For this review, use the dimensioned drawing (mm, ordinates from the lowest corner) and the shaded views. A direction names the side the tool comes from. Give positions to 0.01 mm unless a question says otherwise; leave off trailing zeros. Order: outer loops, then holes, each group sorted by start corner. A loop starts at its lowest first (then second) coordinate and runs counter-clockwise, first axis right, second up.
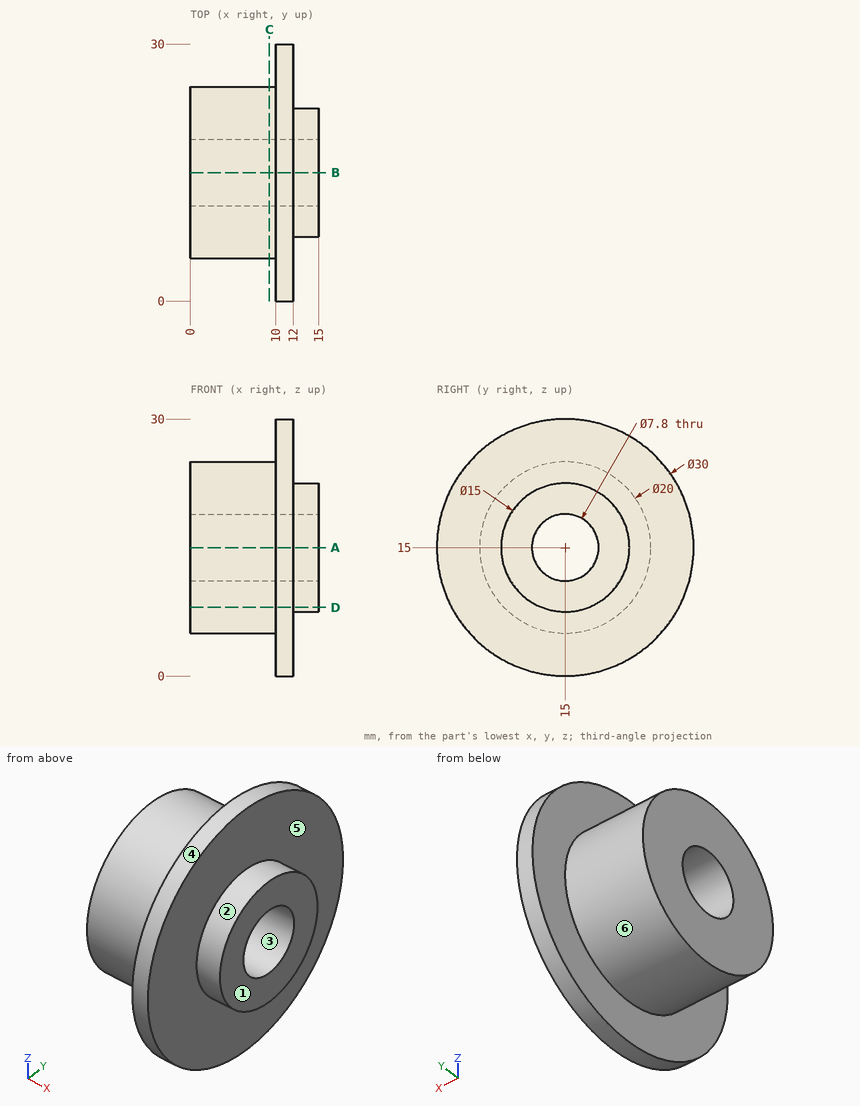
1. Draft analysis for pull direction Z (two halves, no side actions). For the marked faces 1, 2 and 3, state which applies: pulls with the +Z half, pulls with the -Z half, needs draft (parallel to the pull), parting line crosses it, or undercut.
Recorded:
face 1: needs draft
face 2: parting line crosses it
face 3: undercut
2. For line 1 along Z through (x, y) = (3, 15); line 2 along Z through (x, y) = (12.25, 15); line 3 along X through (y, z) = (24.25, 10), list the stretches that pass through material, from the lowest coordinate up.
Recorded:
line 1: z = 5 to 11.1, 18.9 to 25
line 2: z = 7.5 to 11.1, 18.9 to 22.5
line 3: x = 10 to 12
3. Take a section at C-C (x = 9.25). State the section outline as (y, z) points.
Recorded:
outline: circle Ø20 at (15, 15); hole circle Ø7.8 at (15, 15)
4. Machinability: for the marked faces 4, 5 and 6, which of the approach directions +Z, -Z, +X, -X, +Y, -Y give a long, thin tool a straight path to every point of the face, cutting with its end or side? Answer none if there is none.
Recorded:
face 4: +X, -X
face 5: +X
face 6: -X
5. Take a section at D-D (z = 8). State the section outline as (x, y) points, then the cut area to 3 significant figures.
Recorded:
outline: (0, 7.86) - (10, 7.86) - (10, 1.73) - (12, 1.73) - (12, 12.31) - (15, 12.31) - (15, 17.69) - (12, 17.69) - (12, 28.27) - (10, 28.27) - (10, 22.14) - (0, 22.14) - close
area: 212 mm2
6. Take a section at A-A (z = 15). State the section outline as (x, y) points, then the cut area to 3 significant figures.
Recorded:
outline: (0, 5) - (10, 5) - (10, 0) - (12, 0) - (12, 7.5) - (15, 7.5) - (15, 11.1) - (0, 11.1) - close; (0, 18.9) - (15, 18.9) - (15, 22.5) - (12, 22.5) - (12, 30) - (10, 30) - (10, 25) - (0, 25) - close
area: 188 mm2
7. For pin 1 (8 mm diameter, centred on x = 9.5, y = 21.5, fed in from -Z); pin 2 (8 mm diameter, centred on x = 4, z = 27, fed in from -Y); pin 3 (5 mm diameter, centred on x = 4, z = 21, fed in from +Y), all flat-tipped, find the tip position at first contact; note any pin that passes through.
Recorded:
pin 1: stops at z = 0.22
pin 2: stops at y = 9
pin 3: stops at y = 24.37
